Check sheet for the drawn part. Datum: minimum x, y, z corner. Units: mm. Coordinates: 2 decimals unless noted, no trailing zeros. Loops run counter-clockwise (first coordinate to the right, second up) from the corner with the lowest first, then second, coordinate; pieces in that order, holes last.
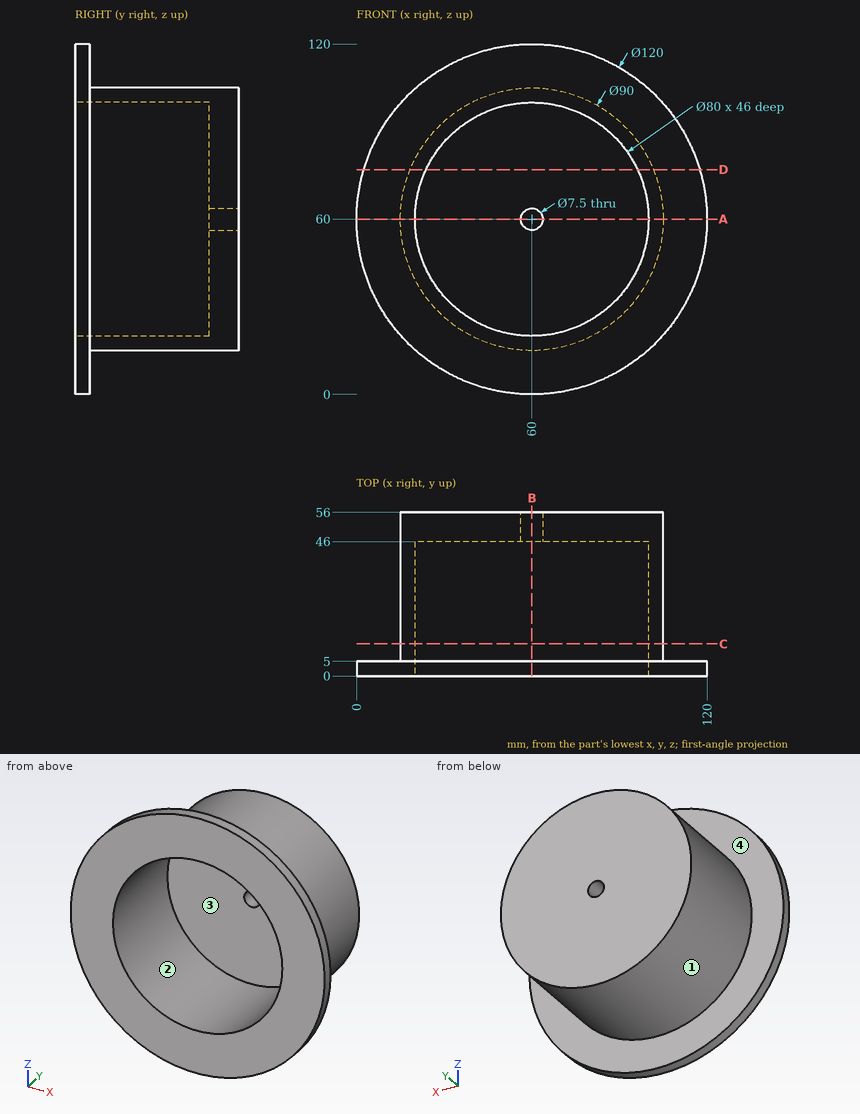
(1) Sectioned sample at C-C on y = 11. Record the cut outline in (x, z).
Findings:
outline: circle Ø90 at (60, 60); hole circle Ø80 at (60, 60)
(2) Scan lines: L1, parallel to Z at x = 60, y = 17; L2, parallel to X at y = 39, z = 61.5 (3 decimals); L3, parallel to X at y = 49.5, z = 60. Record each from-to range of solid material in increasing order.
Findings:
L1: z = 15 to 20, 100 to 105
L2: x = 15.025 to 20.028, 99.972 to 104.975
L3: x = 15 to 56.25, 63.75 to 105
(3) Sectioned sample at A-A on z = 60. Record the cut outline in (x, y), and give its area (4 significant figures).
Findings:
outline: (0, 0) - (20, 0) - (20, 46) - (56.25, 46) - (56.25, 56) - (15, 56) - (15, 5) - (0, 5) - close; (63.75, 46) - (100, 46) - (100, 0) - (120, 0) - (120, 5) - (105, 5) - (105, 56) - (63.75, 56) - close
area: 1,435 mm2
(4) Sectioned sample at D-D on z = 77. Record the cut outline in (x, y).
Findings:
outline: (2.46, 0) - (23.79, 0) - (23.79, 46) - (96.21, 46) - (96.21, 0) - (117.54, 0) - (117.54, 5) - (101.67, 5) - (101.67, 56) - (18.33, 56) - (18.33, 5) - (2.46, 5) - close
(5) Draft check along Z on the marked faces 1, 2, 3 and 4. Enter one of: +Z half, -Z half, draft (parallel to the pull), parting line (faces both ways), or undercut.
Findings:
face 1: parting line
face 2: undercut
face 3: undercut
face 4: draft
(6) Gauge pin test, flat ends, axial feed: pin 1 Ø12 at (x, y) = (24, 15.5) entering from -Z; pin 2 Ø1.5 at (x, y) = (55, 35.5) entering from +Z; pin 3 Ø10 at (x, z) = (60, 60) entering from -Y. Record the tip position at first contact, or that the pin passes through.
Findings:
pin 1: stops at z = 26.46
pin 2: stops at z = 104.8
pin 3: stops at y = 46
(7) Sectioned sample at B-B on x = 60. Record the cut outline in (y, z), and give its area (4 significant figures).
Findings:
outline: (0, 0) - (5, 0) - (5, 15) - (56, 15) - (56, 56.25) - (46, 56.25) - (46, 20) - (0, 20) - close; (0, 100) - (46, 100) - (46, 63.75) - (56, 63.75) - (56, 105) - (5, 105) - (5, 120) - (0, 120) - close
area: 1,435 mm2
